```python
from build123d import *

# Parameters (mm, degrees)
BOSS_EXTRUDE1_DEPTH = 4
SKETCH2_R           = 8
BOSS_EXTRUDE3_DEPTH = 8
SKETCH3_R           = 5
CUT_EXTRUDE2_DEPTH  = 12
SKETCH4_R           = 5
CUT_EXTRUDE3_DEPTH  = 12
SKETCH6_R           = 9.5
BOSS_EXTRUDE6_DEPTH = 1.5
SKETCH15_R          = 5
CUT_EXTRUDE8_DEPTH  = 3.5


with BuildPart() as part:
    # Sketch1 → Boss-Extrude1 (new body)
    with BuildSketch(Plane.XY):
        Polygon((5.675106298, -9.387571669), (10.967428694, 0.221000389), (5.292322396, 9.608572058), (-5.675106298, 9.387571669), (-10.967428694, -0.221000389), (-5.292322396, -9.608572058), align=None)
    boss_extrude1 = extrude(amount=BOSS_EXTRUDE1_DEPTH)

    # Sketch2 → Boss-Extrude3 (add)
    with BuildSketch(Plane.XY.offset(4)):
        Circle(SKETCH2_R)
    boss_extrude3 = extrude(amount=BOSS_EXTRUDE3_DEPTH)

    # Sketch3 → Cut-Extrude2 (cut)
    with BuildSketch(Plane.XY.offset(12)):
        Circle(SKETCH3_R)
    extrude(amount=-CUT_EXTRUDE2_DEPTH, mode=Mode.SUBTRACT)

    # Mirror2: Boss-Extrude1, Boss-Extrude3 across plane
    add(boss_extrude1.mirror(Plane(origin=(0, 0, 2), x_dir=(1, 0, 0), z_dir=(0, 0, -1))))
    add(boss_extrude3.mirror(Plane(origin=(0, 0, 2), x_dir=(1, 0, 0), z_dir=(0, 0, -1))))

    # Sketch4 → Cut-Extrude3 (cut)
    with BuildSketch(Plane(origin=(0, 0, -8), x_dir=(-1, 0, 0), z_dir=(0, 0, -1))):
        Circle(SKETCH4_R)
    extrude(amount=-CUT_EXTRUDE3_DEPTH, mode=Mode.SUBTRACT)

    # Sketch6 → Boss-Extrude6 (add)
    with BuildSketch(Plane.XY.offset(4)):
        Circle(SKETCH6_R)
    extrude(amount=BOSS_EXTRUDE6_DEPTH)

    # Sketch15 → Cut-Extrude8 (cut)
    with BuildSketch(Plane.XY.offset(4)):
        Circle(SKETCH15_R)
    extrude(amount=CUT_EXTRUDE8_DEPTH, mode=Mode.SUBTRACT)


solid = part.part
```
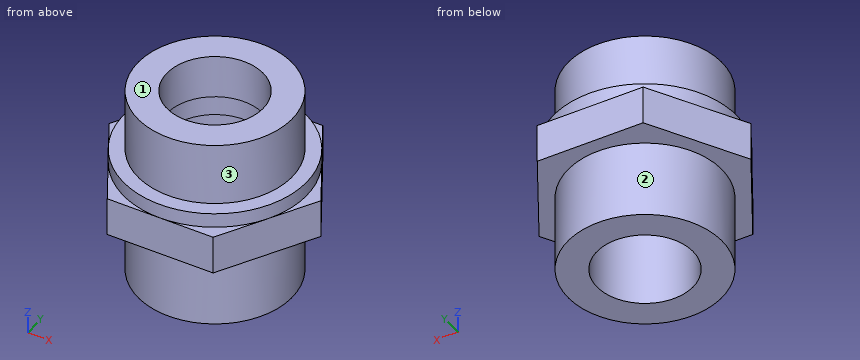
Could you check a few things on this model? Use its own coordinates, in mm. Face numbers are marked on the shaded views. A direction names the side the tool comes from. Give positions to 0.01 mm unless a question says otherwise; leave off trailing zeros. Loops run counter-clockwise (first coordinate to the right, second up) from the corner with the lowest first, then second, coordinate; pieces in that order, holes last. Notation, with made-up numbers: (-28, -10) - (-22, -10) arc R29 ccw to (-22, 19) - close; hole circle Ø4 at (-31, 39). An arc over 180 degrees is marked (long way). Use one line per item in the form item = value.
1. I want a section at C-C (y = -1.5). Please give me the cut outline in (x, z), and give its area (3 significant figures).
Response values:
outline = (-10.19, 0) - (-7.86, 0) - (-7.86, -8) - (-4.77, -8) - (-4.77, 12) - (-7.86, 12) - (-7.86, 5.5) - (-9.38, 5.5) - (-9.38, 4) - (-10.19, 4) - close; (4.77, -8) - (7.86, -8) - (7.86, 0) - (10.02, 0) - (10.02, 4) - (9.38, 4) - (9.38, 5.5) - (7.86, 5.5) - (7.86, 12) - (4.77, 12) - close
area = 146 mm²
2. I want a section at D-D (x = 7.5). Please give me the cut outline in (y, z), and give its area (3 significant figures).
Response values:
outline = (-6.07, 0) - (-2.78, 0) - (-2.78, -8) - (2.78, -8) - (2.78, 0) - (5.96, 0) - (5.96, 4) - (5.83, 4) - (5.83, 5.5) - (2.78, 5.5) - (2.78, 12) - (-2.78, 12) - (-2.78, 5.5) - (-5.83, 5.5) - (-5.83, 4) - (-6.07, 4) - close
area = 146 mm²
3. I'm going to push flat-ended pins straight in: pin 1 Ø1.4 at (x, y) = (9, -1.5) entering from +Z; pin 2 Ø1.5 at (y, z) = (-4, 2.5) entering from +X; pin 3 Ø3 at (x, z) = (6.5, 10) entering from -Y (3 decimals). Where does each tip first touch, or does it pass through?
Response values:
pin_1 = 5.5
pin_2 = 9.06
pin_3 = -6.245
4. I want a section at B-B (z = 2). Please give me the cut outline in (x, y), and give its area (3 significant figures).
Response values:
outline = (-10.97, -0.22) - (-5.29, -9.61) - (5.68, -9.39) - (10.97, 0.22) - (5.29, 9.61) - (-5.68, 9.39) - close; hole circle Ø10 at (0, 0)
area = 234 mm²
5. On a 3-axis mill with a long thin cutter (end or side, diameter ignored), from which of +Z, -Z, +X, -X, +Y, -Y can I reach the whole of each face in a straight line? I mean the marked faces 1, 2 and 3. Say none if no direction works.
Response values:
face_1 = +Z, +X, -X, +Y, -Y
face_2 = -Z
face_3 = +Z
6. I need wall thicknesses on probe 1 along X at (y, z) = (0, 5.05); probe 2 along Y at (x, z) = (0, 6.3). Which ranges of each line are inside material? Lowest first, please.
Response values:
probe_1 = -9.5 to -5, 5 to 9.5
probe_2 = -8 to -5, 5 to 8
